```python
from build123d import *

# Parameters (mm, degrees)
SKETCH2_R           = 12.7
SKETCH2_R_2         = 1.077000005
BOSS_EXTRUDE1_DEPTH = 3.175
SKETCH3_W           = 9.017
SKETCH3_H           = 9.017
BOSS_EXTRUDE2_DEPTH = 19.05
SKETCH4_R           = 3.175
CUT_EXTRUDE1_DEPTH  = 58.957935729


with BuildPart() as part:
    # Sketch2 → Boss-Extrude1 (new, symmetric)
    # profile 1 of 2: a face of its own
    with BuildSketch(Plane.XY):
        with BuildLine():
            Line((25.4, 47.117), (16.383, 47.117))
            Line((16.383, 47.117), (16.383, 12.7))
            Line((16.383, 12.7), (0, 12.7))
            ThreePointArc((0, 12.7), (8.980256121, 8.980256121), (12.7, 0))
            ThreePointArc((12.7, 0), (8.980256121, -8.980256121), (0, -12.7))
            Line((0, -12.7), (25.4, -12.7))
            Line((25.4, -12.7), (25.4, 47.117))
        make_face()
    # profile 2 of 2: a face of its own
    with BuildSketch(Plane.XY):
        Circle(SKETCH2_R)
        with Locations((0, 6.99999997)):
            Circle(SKETCH2_R_2, mode=Mode.SUBTRACT)
        with Locations((-6.99999997, 0)):
            Circle(SKETCH2_R_2, mode=Mode.SUBTRACT)
        with Locations((0, -6.99999997)):
            Circle(SKETCH2_R_2, mode=Mode.SUBTRACT)
        with Locations((6.99999997, 0)):
            Circle(SKETCH2_R_2, mode=Mode.SUBTRACT)
    extrude(amount=BOSS_EXTRUDE1_DEPTH, both=True)

    # Sketch3 → Boss-Extrude2 (add, symmetric)
    with BuildSketch(Plane(origin=(0, 0, 0), x_dir=(-1, 0, 0), z_dir=(0, 0, -1))):
        with Locations((-20.8915, 42.6085)):
            Rectangle(SKETCH3_W, SKETCH3_H)
    extrude(amount=BOSS_EXTRUDE2_DEPTH, both=True)

    # Sketch4 → Cut-Extrude1 (cut, through all)
    with BuildSketch(Plane.XY.offset(3.175)):
        Circle(SKETCH4_R)
    extrude(amount=-CUT_EXTRUDE1_DEPTH, mode=Mode.SUBTRACT)


solid = part.part
```
Geometry: final body of the model. Coordinates: model frame, mm. A direction names the side the tool comes from. Round coordinates to 2 decimals unless told otherwise and drop trailing zeros. Order: outer loops, then holes, each group sorted by start corner. A loop starts at its lowest first (then second) coordinate and runs counter-clockwise, first axis right, second up. Notation, with made-up numbers: (41.5, 73) -> (58.5, 73) arc R15 ccw to (58.5, 97) -> close; hole circle Ø6 at (-1.75, -30.75). An arc over 180 degrees is marked (long way). Use one line per item in the form item = value. Start each with the question number.
1. Line query: probe 1 along Z at (x, y) = (17, 10.5) (3 decimals); probe 2 along X at (y, z) = (42, -7); probe 3 along Y at (x, z) = (24.5, -8.5). Output: solid intervals per line, ascending.
2. Cut plane C-C (x = -7). Return the cut outline in (y, z) (3 decimals).
3. Cut plane A-A (y = 0). Return the cut outline in (x, z) (3 decimals), then the cut area to 3 significant figures.
4. Cut plane B-B (x = 23). Return the cut outline in (y, z) (3 decimals).
5. Draft query along X for faces 1 (the face through (8, -0.4, 0)), 2 (the face through (25.4, 26, 0)), 3 (the face through (13, -12.7, 0)). Return one class per face: pulls with the +X half, pulls with the -X half, needs draft (parallel to the pull), parting line crosses it, or undercut.
6. Cut plane D-D (y = -7). Return the cut outline in (x, z) (3 decimals).
7. Reachability of faces 4 (the face through (-0.233, 5.949, -0.044)), 5 (the face through (10, 7, 3.175)), 6 (the face through (10, 7, -3.175)), 7 (the face through (16.383, 37, 0)) from +Z, -Z, +X, -X, +Y, -Y: full face, straight path, thin tool, end or side. Return the list, or none.
8. Pin query (flat end, axial travel): pin 1 Ø6 at (x, y) = (17.5, 21) entering from -Z (3 decimals); pin 2 Ø10 at (y, z) = (12.5, -9) entering from -X; pin 3 Ø2.5 at (x, z) = (21, -11.5) entering from -Y; pin 4 Ø1.9 at (x, z) = (5.5, -1) entering from +Y. Return the tip coordinate at first contact, or that it passes through.
Solution:
q1.probe_1 = -3.175 to 3.175
q1.probe_2 = 16.38 to 25.4
q1.probe_3 = 38.1 to 47.12
q2.outline = (-10.597, -3.175) -> (-1.077, -3.175) -> (-1.077, 3.175) -> (-10.597, 3.175) -> close; (1.077, -3.175) -> (10.597, -3.175) -> (10.597, 3.175) -> (1.077, 3.175) -> close
q3.outline = (-12.7, -3.175) -> (-8.077, -3.175) -> (-8.077, 3.175) -> (-12.7, 3.175) -> close; (-5.923, -3.175) -> (-3.175, -3.175) -> (-3.175, 3.175) -> (-5.923, 3.175) -> close; (3.175, -3.175) -> (5.923, -3.175) -> (5.923, 3.175) -> (3.175, 3.175) -> close; (8.077, -3.175) -> (25.4, -3.175) -> (25.4, 3.175) -> (8.077, 3.175) -> close
q3.area = 174 mm^2
q4.outline = (-12.7, -3.175) -> (38.1, -3.175) -> (38.1, -19.05) -> (47.117, -19.05) -> (47.117, 19.05) -> (38.1, 19.05) -> (38.1, 3.175) -> (-12.7, 3.175) -> close
q5.face_1 = undercut
q5.face_2 = pulls with the +X half
q5.face_3 = needs draft
q6.outline = (-10.597, -3.175) -> (-1.077, -3.175) -> (-1.077, 3.175) -> (-10.597, 3.175) -> close; (1.077, -3.175) -> (25.4, -3.175) -> (25.4, 3.175) -> (1.077, 3.175) -> close
q7.face_4 = +Z, -Z
q7.face_5 = +Z, +X, -X, -Y
q7.face_6 = -Z, +X, -X, -Y
q7.face_7 = +Z, -Z, -X, +Y
q8.pin_1 = -3.175
q8.pin_2 = through
q8.pin_3 = 38.1
q8.pin_4 = 12.7
